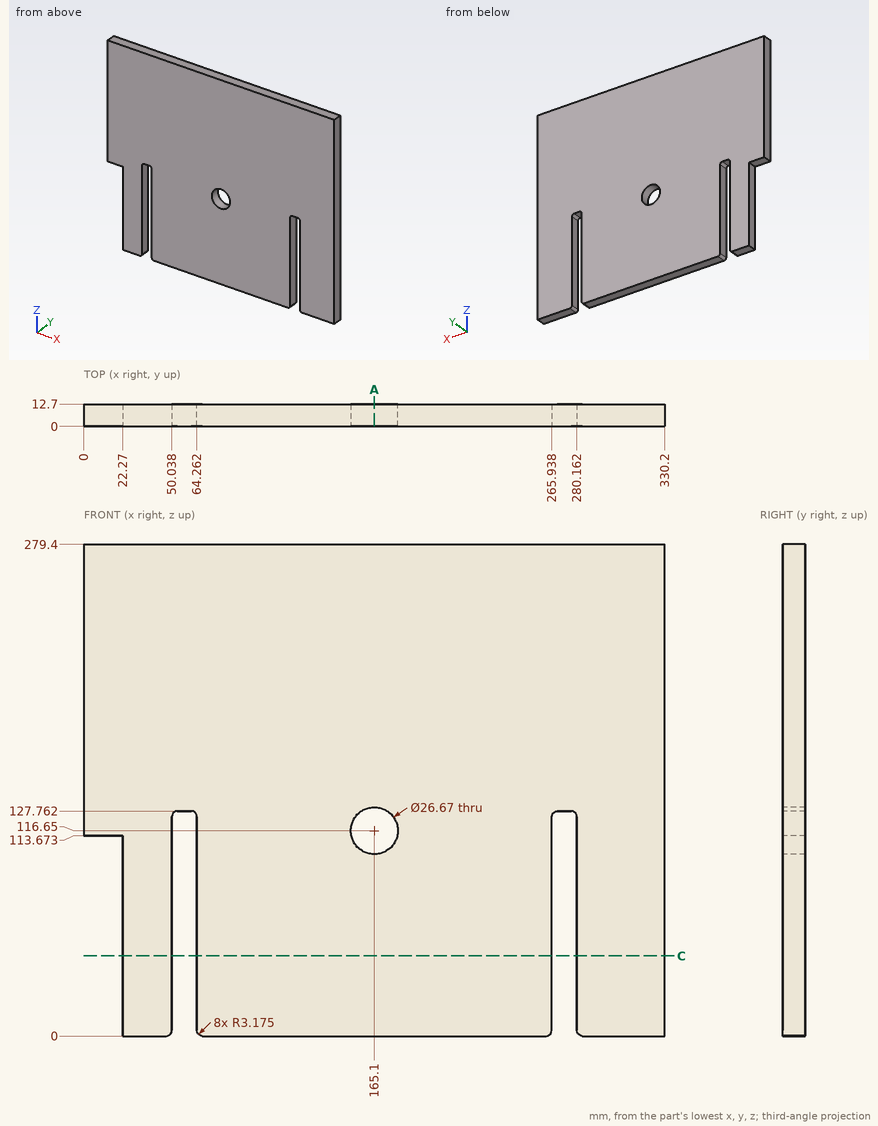
Geometry: see drawing. Coordinates: mm, zero at the bounding-box minimum. Round coordinates to 2 decimals unless told otherwise and drop trailing zeros. Loops run counter-clockwise (first coordinate to the right, second up) from the corner with the lowest first, then second, coordinate; pieces in that order, holes last. Notation, with made-up numbers: (20, -32) - (26, -32) arc R10 cw to (26, -15) - close; hole circle Ø7 at (46.25, 22.25). An arc over 180 degrees is marked (long way). Use CSV: the item, a comma, the result in double quotes.
Q1. Section query A-A, the plane x = 165.1. Output: boundary loops of the cut face in (y, z) (1 decimal), then the cut area to 3 significant figures.
Reported:
outline,"(0, 0) - (12.7, 0) - (12.7, 103.3) - (0, 103.3) - close; (0, 130) - (12.7, 130) - (12.7, 279.4) - (0, 279.4) - close"
area,"3,210 mm^2"
Q2. Ray query, line 1 along X through (y, z) = (8, 116.65) (1 decimal); line 2 along X through (y, z) = (4.5, 50); line 3 along Z through (x, y) = (165.1, 3) (1 decimal). Return the intervals inside material, ascending.
Reported:
line 1,"0 to 50, 64.3 to 151.8, 178.4 to 265.9, 280.2 to 330.2"
line 2,"22.27 to 50.04, 64.26 to 265.94, 280.16 to 330.2"
line 3,"0 to 103.3, 130 to 279.4"
Q3. Section query C-C, the plane z = 45.5. Output: boundary loops of the cut face in (x, y), then the cut area to 3 significant figures.
Reported:
outline,"(22.27, 0) - (50.04, 0) - (50.04, 12.7) - (22.27, 12.7) - close; (64.26, 0) - (265.94, 0) - (265.94, 12.7) - (64.26, 12.7) - close; (280.16, 0) - (330.2, 0) - (330.2, 12.7) - (280.16, 12.7) - close"
area,"3,550 mm^2"
Q4. Pin query (flat end, axial travel): pin 1 Ø1.5 at (x, z) = (106, 85) entering from -Y; pin 2 Ø4 at (x, y) = (273, 3.5) entering from -Z; pin 3 Ø6.5 at (y, z) = (7.5, 43.5) entering from -X. Return the tip coordinate at first contact, or that it passes through.
Reported:
pin 1,"y = 0"
pin 2,"z = 127.76"
pin 3,"x = 22.27"
